Verification items for this drawing (mm, ordinates from the low corner). A direction names the side the tool comes from. Round coordinates to 2 decimals unless told otherwise and drop trailing zeros. Order: outer loops, then holes, each group sorted by start corner. A loop starts at its lowest first (then second) coordinate and runs counter-clockwise, first axis right, second up.
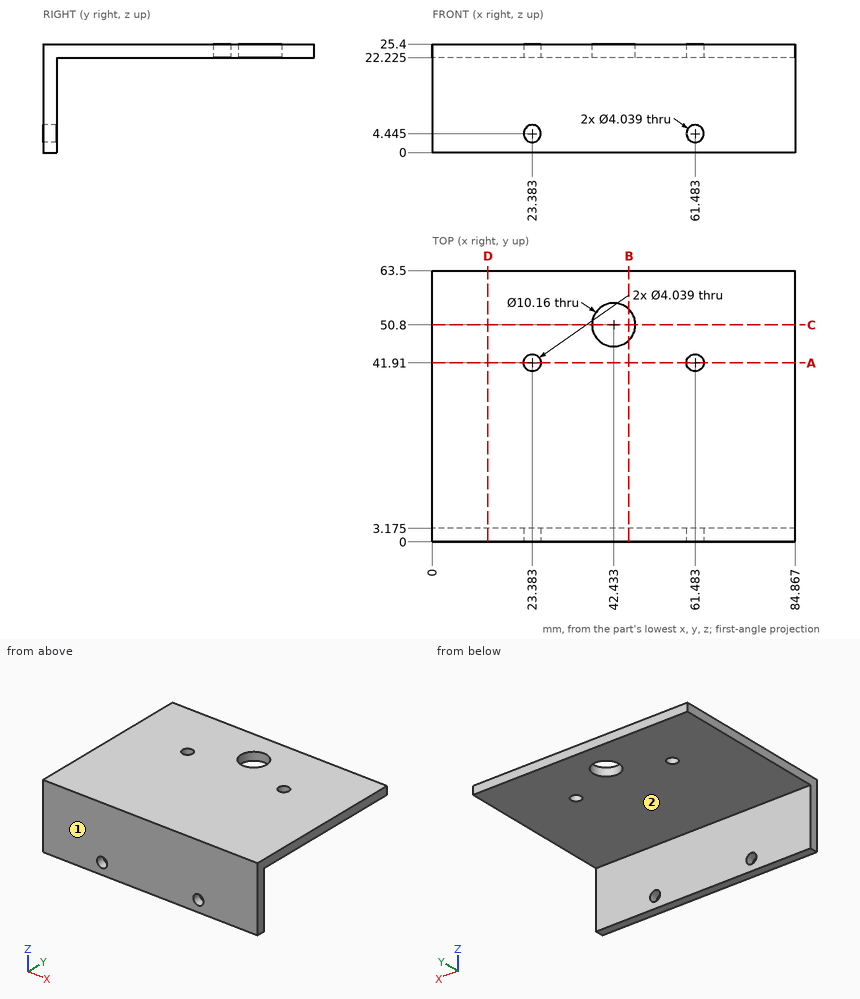
Item 1: Sectioned sample at B-B (x = 46). Record the cut outline in (y, z) (1 decimal), and give its area (3 significant figures).
Answer:
outline: (0, 0) - (3.2, 0) - (3.2, 22.2) - (47.2, 22.2) - (47.2, 25.4) - (0, 25.4) - close; (54.4, 22.2) - (63.5, 22.2) - (63.5, 25.4) - (54.4, 25.4) - close
area: 249 mm2
Item 2: Sectioned sample at D-D (x = 13). Record the cut outline in (y, z) (1 decimal), and give its area (3 significant figures).
Answer:
outline: (0, 0) - (3.2, 0) - (3.2, 22.2) - (63.5, 22.2) - (63.5, 25.4) - (0, 25.4) - close
area: 272 mm2
Item 3: Access from +Z, -Z, +X, -X, +Y, -Y to the whole of each face (thin tool, end or side, straight path). Record for the marked faces 1 and 2.
Answer:
face 1: +Z, -Z, +X, -X, -Y
face 2: -Z, +X, -X, +Y
Item 4: Sectioned sample at A-A (y = 41.91). Record the cut outline in (x, z) (1 decimal).
Answer:
outline: (0, 22.2) - (21.4, 22.2) - (21.4, 25.4) - (0, 25.4) - close; (25.4, 22.2) - (59.5, 22.2) - (59.5, 25.4) - (25.4, 25.4) - close; (63.5, 22.2) - (84.9, 22.2) - (84.9, 25.4) - (63.5, 25.4) - close
Item 5: Scan lines: line 1 along Y through (x, z) = (66.5, 2.5) (1 decimal); line 2 along Z through (x, y) = (6, 46) (1 decimal). Record each from-to range of solid material in increasing order.
Answer:
line 1: y = 0 to 3.2
line 2: z = 22.2 to 25.4
Item 6: Go/stop test with flat-tipped pins: P1, Ø13, axis at x = 42.43, y = 50.8, coming from the -Z side (3 decimals); P2, Ø10, axis at x = 29, z = 8.5, coming from the +Y side (3 decimals). Record where each tip stops, or that it passes through.
Answer:
P1: stops at z = 22.225
P2: stops at y = 3.175
Item 7: Sectioned sample at C-C (y = 50.8). Record the cut outline in (x, z) (1 decimal), and give its area (3 significant figures).
Answer:
outline: (0, 22.2) - (37.4, 22.2) - (37.4, 25.4) - (0, 25.4) - close; (47.5, 22.2) - (84.9, 22.2) - (84.9, 25.4) - (47.5, 25.4) - close
area: 237 mm2
